```python
from build123d import *

# Parameters (mm, degrees)
SKETCH1_R           = 31.75
BOSS_EXTRUDE1_DEPTH = 698.5
SKETCH2_R           = 31.75
BOSS_EXTRUDE2_DEPTH = 63.5
SKETCH3_R           = 31.75
BOSS_EXTRUDE3_DEPTH = 63.5
CUT_EXTRUDE1_DEPTH  = 63.5


with BuildPart() as part:
    # Sketch1 → Boss-Extrude1 (new body)
    with BuildSketch(Plane(origin=(0, 0, 0), x_dir=(1, 0, 0), z_dir=(0, 1, 0))):
        Circle(SKETCH1_R)
    extrude(amount=BOSS_EXTRUDE1_DEPTH)

    # Sketch2 → Boss-Extrude2 (add)
    with BuildSketch(Plane(origin=(0, 698.5, 0), x_dir=(1, 0, 0), z_dir=(0, 1, 0))):
        Circle(SKETCH2_R)
    extrude(amount=BOSS_EXTRUDE2_DEPTH)

    # Sketch3 → Boss-Extrude3 (add)
    with BuildSketch(Plane.XZ):
        Circle(SKETCH3_R)
    extrude(amount=BOSS_EXTRUDE3_DEPTH)

    # Sketch4 → Cut-Extrude1 (cut)
    with BuildSketch(Plane(origin=(31.75, 0, 0), x_dir=(0, 0, -1), z_dir=(1, 0, 0))):
        Polygon((-31.75, 762), (-31.75, 698.5), (31.75, 762), align=None)
        Polygon((-31.75, 0), (31.75, -63.5), (-31.75, -63.5), align=None)
    extrude(amount=-CUT_EXTRUDE1_DEPTH, mode=Mode.SUBTRACT)


solid = part.part
```
Check sheet for the modelled part. Datum: model origin and axes. Units: mm. Give positions to 0.01 mm unless a question says otherwise; leave off trailing zeros. Loops run counter-clockwise (first coordinate to the right, second up) from the corner with the lowest first, then second, coordinate; pieces in that order, holes last. Notation, with made-up numbers: M -31.5,50 L 14.5,50 A17 cw 14.5,83 Z; hole C 28,-32.75 d6. An arc over 180 degrees is marked long. Answer as CSV lines item,"result".
Item 1: Sectioned sample at D-D, the plane y = -13. Enter the section's corners in (x, z), then the cut area to 3 significant figures.
Reply:
outline,"M -25.62,18.75 A31.75 ccw long 25.62,18.75 Z"
area,"2,700 mm^2"
Item 2: Sectioned sample at B-B, the plane z = 0. Enter the section's corners in (x, y).
Reply:
outline,"M -31.75,-31.75 L 31.75,-31.75 L 31.75,730.25 L -31.75,730.25 Z"
Item 3: Depth check by flat-ended pin: pin 1 Ø12 at (x, y) = (16.5, 653) entering from +Z; pin 2 Ø10 at (x, y) = (-12.5, 73.5) entering from -Z; pin 3 Ø4 at (x, z) = (-16, -21.5) entering from -Y; pin 4 Ø5 at (x, y) = (-1.5, 297.5) entering from -Z. Enter the tip coordinate at first touch or a pass-through.
Reply:
pin 1,"z = 29.96"
pin 2,"z = -30.85"
pin 3,"y = -55.25"
pin 4,"z = -31.75"
Item 4: Scan lines: L1, parallel to X at y = 453, z = 1.5; L2, parallel to X at y = 166, z = 2.5. Record each from-to range of solid material in increasing order.
Reply:
L1,"-31.71 to 31.71"
L2,"-31.65 to 31.65"
Item 5: Sectioned sample at A-A, the plane x = 0. Enter the section's corners in (y, z), then the cut area to 3 significant figures.
Reply:
outline,"M -63.5,-31.75 L 762,-31.75 L 698.5,31.75 L 0,31.75 Z"
area,"48,400 mm^2"
Item 6: Sectioned sample at C-C, the plane y = 504.5. Enter the section's corners in (x, z).
Reply:
outline,"C 0,0 d63.5"
